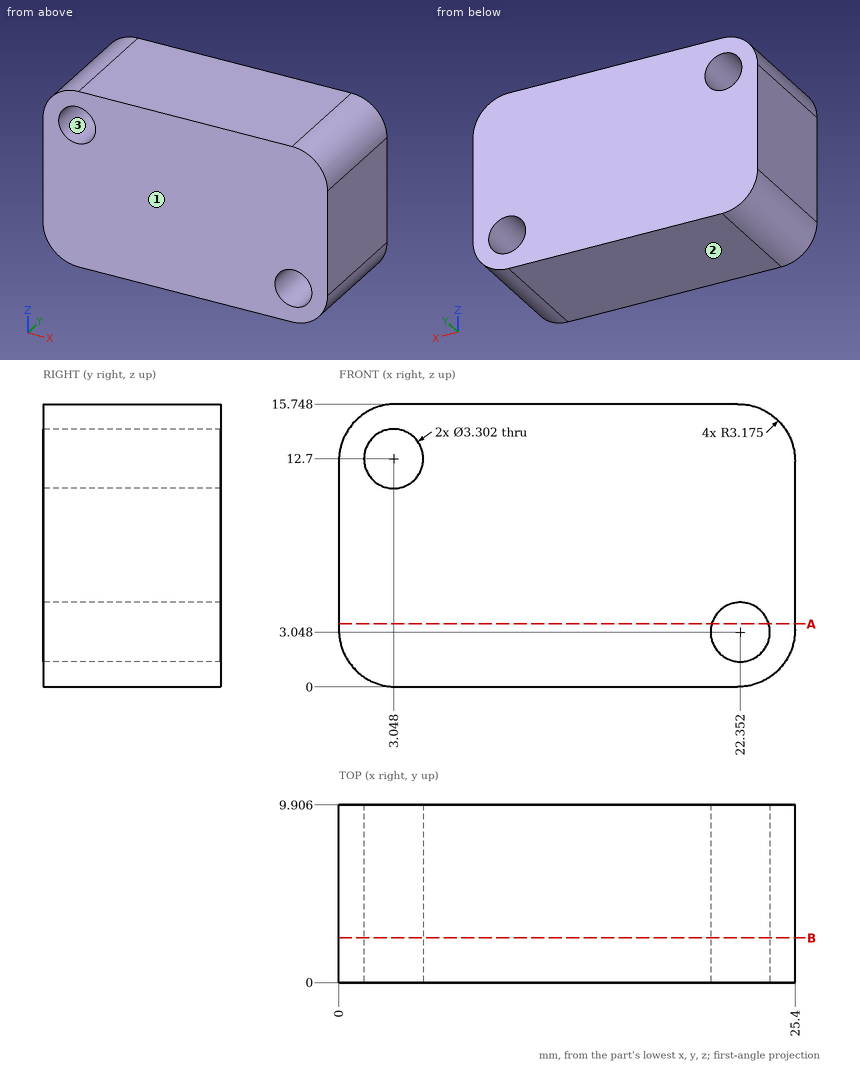
Verification items for this drawing (mm, ordinates from the low corner). Give positions to 0.01 mm unless a question says otherwise; leave off trailing zeros. Loops run counter-clockwise (first coordinate to the right, second up) from the corner with the lowest first, then second, coordinate; pieces in that order, holes last. Notation, with made-up numbers: M 85,15.5 L 90,15.5 A34 cw 90,52.5 Z; hole C 52,-28.75 d9. An arc over 180 degrees is marked long. Answer as a JSON object with one key per item and string values. Group by question number.
Item 1: Sectioned sample at B-B on y = 2.5. Record the boundary of the cut face in (x, z) (3 decimals).
Item 2: Mould release check, pull along Z, two halves, no side actions. Record for the marked faces 1, 2 and 3: pulls with the +Z half, pulls with the -Z half, needs draft (parallel to the pull), parting line crosses it, or undercut.
Item 3: Sectioned sample at A-A on z = 3.5. Record the boundary of the cut face in (x, y).
Item 4: Material ranges on L1, parallel to X at y = 4.5, z = 12.7; L2, parallel to X at y = 9, z = 3; L3, parallel to X at y = 8.75, z = 15.25, recorded low to high.
Findings below:
{
 "1": {"outline": "M 0,3.175 A3.175 ccw 3.175,0 L 22.225,0 A3.175 ccw 25.4,3.175 L 25.4,12.573 A3.175 ccw 22.225,15.748 L 3.175,15.748 A3.175 ccw 0,12.573 Z; hole C 3.048,12.7 d3.302; hole C 22.352,3.048 d3.302"},
 "2": {"face 1": "needs draft", "face 2": "pulls with the -Z half", "face 3": "undercut"},
 "3": {"outline": "M 0,0 L 20.76,0 L 20.76,9.91 L 0,9.91 Z; M 23.94,0 L 25.4,0 L 25.4,9.91 L 23.94,9.91 Z"},
 "4": {"L1": "0 to 1.4, 4.7 to 25.4", "L2": "0 to 20.7, 24 to 25.4", "L3": "1.47 to 23.93"}
}
